Could you check a few things on this drawing? It's one solid part, dimensions in mm from its lowest x, y, z. A direction names the side the tool comes from. Round coordinates to 2 decimals unless told otherwise and drop trailing zeros. Write each loop counter-clockwise with the first axis right and the second up, starting at its lowest first coordinate (ties: lowest second). Pieces come first, ordered by that corner, then holes. Notation, with made-up numbers: (49, 56.5) -> (66, 56.5) arc R26 cw to (66, 90.5) -> close; hole circle Ø6 at (64.25, 77). An arc over 180 degrees is marked (long way). Answer as CSV lines item,"result".
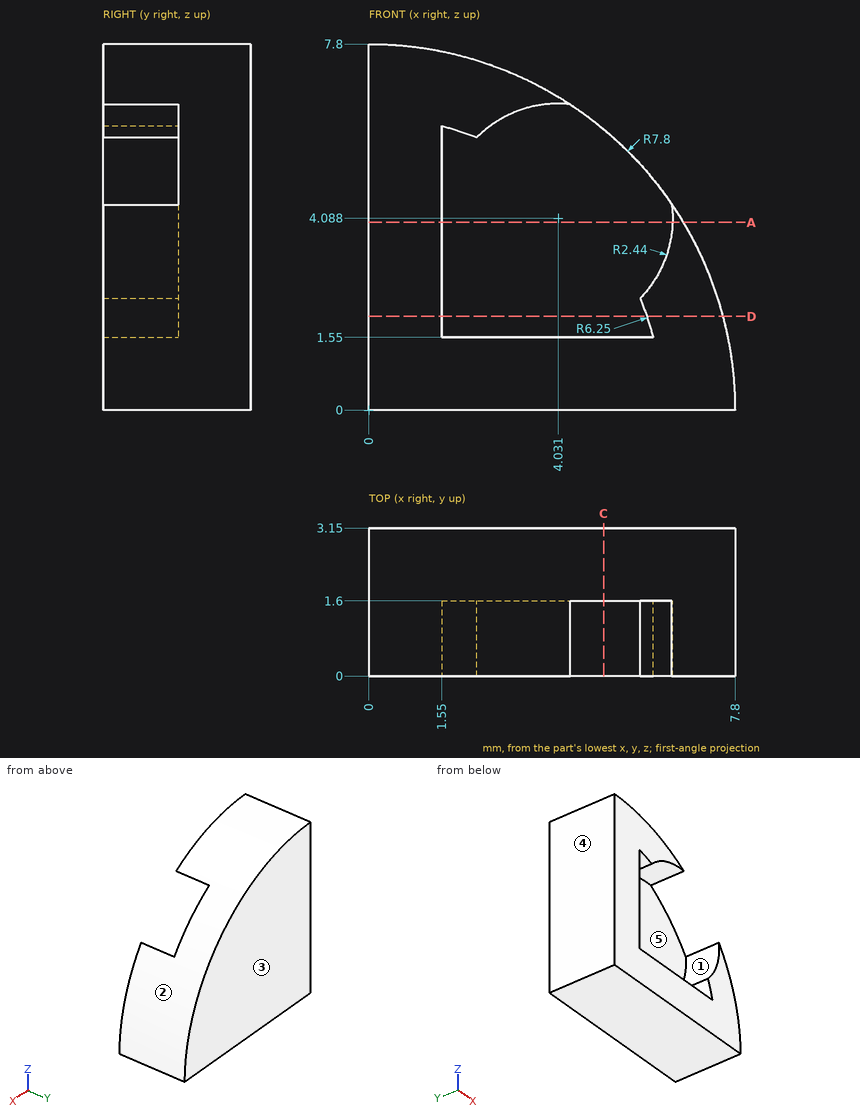
1. Suppose I cut it at A-A on z = 4. Please give me the cut outline in (x, y), and give its area (3 significant figures).
Numbers:
outline,"(0, 0) -> (1.55, 0) -> (1.55, 1.6) -> (6.47, 1.6) -> (6.47, 0) -> (6.7, 0) -> (6.7, 3.15) -> (0, 3.15) -> close"
area,"13.2 mm^2"
2. If we mould it in two halves opening along Z, with no side actions, what happens to the marked faces 1, 2 and 3? For each: released by +Z, released by -Z, zero draft, split by the parting line, or undercut.
Numbers:
face 1,"undercut"
face 2,"released by +Z"
face 3,"zero draft"
3. Suppose I cut it at C-C on x = 5. Please give me the cut outline in (y, z).
Numbers:
outline,"(0, 0) -> (3.15, 0) -> (3.15, 5.99) -> (1.6, 5.99) -> (1.6, 1.55) -> (0, 1.55) -> close"
4. On a 3-axis mill with a long thin cutter (end or side, diameter ignored), from which of +Z, -Z, +X, -X, +Y, -Y can I reach the whole of each face in a straight line? I mean the marked faces 4 and 5. Say none if no direction works.
Numbers:
face 4,"+Z, -Z, -X, +Y, -Y"
face 5,"-Y"
5. If I drill on line 1 (Y direction, x = 6, z = 3.75); line 2 (X direction, y = 0.5, z = 2.25); line 3 (X direction, y = 0.8, z = 5.75), over which ranges is the centre line in solid material (lowest first)?
Numbers:
line 1,"y = 1.6 to 3.15"
line 2,"x = 0 to 1.55, 5.83 to 7.47"
line 3,"x = 0 to 1.55"
6. Suppose I cut it at D-D on z = 2. Please give me the cut outline in (x, y).
Numbers:
outline,"(0, 0) -> (1.55, 0) -> (1.55, 1.6) -> (5.92, 1.6) -> (5.92, 0) -> (7.54, 0) -> (7.54, 3.15) -> (0, 3.15) -> close"
7. For pin 1 Ø1.3 at (x, y) = (4, 0.5) entering from +Z (1 decimal); pin 2 Ø1.3 at (y, z) = (0.5, 5) entering from +X (1 decimal), each with a flat end and sliding along its axis, tell me the tip position at first contact or that it passes through.
Numbers:
pin 1,"stops at z = 7"
pin 2,"stops at x = 6.5"
